Check sheet for the modelled part. Datum: model origin and axes. Units: mm. Coordinates: 2 decimals unless noted, no trailing zeros. Order: outer loops, then holes, each group sorted by start corner. A loop starts at its lowest first (then second) coordinate and runs counter-clockwise, first axis right, second up.
1. Gauge pin test, flat ends, axial feed: pin 1 Ø2.5 at (x, z) = (-43.3, -38.4) entering from -Y; pin 2 Ø1 at (x, y) = (76, 1) entering from -Z; pin 3 Ø6.5 at (x, z) = (56.5, 35.5) entering from +Y; pin 4 Ø1 at (x, y) = (14.5, 2.5) entering from +Z. Record the tip position at first contact, or that the pin passes through.
2. Draft check along X on faces 1 (the cylindrical face through (60.84, 1.52, -81.95)), 2 (the flat face through (1, 3, -11)), 3 (the conical face through (-51.97, 2.3, 55.43)). Enter one of: released by +X, released by -X, zero draft, split by the parting line, or undercut.
3. Cross-section at B-B (x = -69.5). Enter the section's corners in (y, z), then the cut area to 3 significant figures.
4. Cross-section at A-A (z = -63.5). Enter the section's corners in (x, y), then the cut area to 3 significant figures.
5. Thickness scan on line 1 (X direction, y = 0.3, z = 3.9); line 2 (X direction, y = 0.3, z = -22); line 3 (X direction, y = 0.3, z = -35.5). Record the ranges inside material, lowest first.
```python
from build123d import *

# Parameters (mm, degrees)
SKETCH1_R                                      = 100
BOSS_EXTRUDE1_DEPTH                            = 3
CSK_FOR_M5_SFHCS1_AT_2_COUNT                   = 2
CSK_FOR_M5_SFHCS1_AT_2_PITCH                   = 23.5
CSK_FOR_M5_SFHCS1_AT_3_COUNT                   = 2
CSK_FOR_M5_SFHCS1_AT_3_PITCH                   = 40.703193978
CSK_FOR_M5_SFHCS1_AT_4_COUNT                   = 2
CSK_FOR_M5_SFHCS1_AT_4_PITCH                   = 47
CSK_FOR_M5_SFHCS1_AT_5_COUNT                   = 2
CSK_FOR_M5_SFHCS1_AT_5_PITCH                   = 40.703193978
CSK_FOR_M5_SFHCS1_AT_6_COUNT                   = 2
CSK_FOR_M5_SFHCS1_AT_6_PITCH                   = 23.5
BOSS_EXTRUDE2_DEPTH                            = 3
FILLET1_R                                      = 20
CSK_FOR_M5_SFHCS2_AT_2_COUNT                   = 2
CSK_FOR_M5_SFHCS2_AT_2_PITCH                   = 35
CSK_FOR_M5_SFHCS2_AT_3_COUNT                   = 2
CSK_FOR_M5_SFHCS2_AT_3_PITCH                   = 45
CSK_FOR_M5_SFHCS2_AT_4_COUNT                   = 2
CSK_FOR_M5_SFHCS2_AT_4_PITCH                   = 57.008771255
CSK_FOR_M5_FLAT_HEAD_MACHINE_SCREW2_AT_2_COUNT = 2
CSK_FOR_M5_FLAT_HEAD_MACHINE_SCREW2_AT_2_PITCH = 70
CSK_FOR_M5_FLAT_HEAD_MACHINE_SCREW2_AT_3_COUNT = 2
CSK_FOR_M5_FLAT_HEAD_MACHINE_SCREW2_AT_3_PITCH = 99.704563587
CSK_FOR_M5_FLAT_HEAD_MACHINE_SCREW2_AT_4_COUNT = 2
CSK_FOR_M5_FLAT_HEAD_MACHINE_SCREW2_AT_4_PITCH = 71
CSK_FOR_M4_FLAT_HEAD_MACHINE_SCREW1_AT_2_COUNT = 2
CSK_FOR_M4_FLAT_HEAD_MACHINE_SCREW1_AT_2_PITCH = 42.3
CSK_FOR_M4_FLAT_HEAD_MACHINE_SCREW1_AT_3_COUNT = 2
CSK_FOR_M4_FLAT_HEAD_MACHINE_SCREW1_AT_3_PITCH = 40.4
CSK_FOR_M4_FLAT_HEAD_MACHINE_SCREW1_AT_4_COUNT = 2
CSK_FOR_M4_FLAT_HEAD_MACHINE_SCREW1_AT_4_PITCH = 58.493161994
CSK_FOR_M5_FLAT_HEAD_MACHINE_SCREW3_AT_2_COUNT = 2
CSK_FOR_M5_FLAT_HEAD_MACHINE_SCREW3_AT_2_PITCH = 155
CSK_FOR_M5_FLAT_HEAD_MACHINE_SCREW3_AT_3_COUNT = 2
CSK_FOR_M5_FLAT_HEAD_MACHINE_SCREW3_AT_3_PITCH = 109.601551084
CSK_FOR_M5_FLAT_HEAD_MACHINE_SCREW3_AT_4_COUNT = 2
CSK_FOR_M5_FLAT_HEAD_MACHINE_SCREW3_AT_4_PITCH = 109.601551084


with BuildPart() as part:
    # Sketch1 → Boss-Extrude1 (new body)
    with BuildSketch(Plane(origin=(0, 0, 0), x_dir=(1, 0, 0), z_dir=(0, 1, 0))):
        with Locations(Location((0, 0, 0), (0, 0, 270))):
            Circle(SKETCH1_R)
    extrude(amount=BOSS_EXTRUDE1_DEPTH)

    # Sketch6 → CSK for M5 SFHCS1 (revolve, cut)
    with BuildSketch(Plane(origin=(-13.325081846, 0, -19.356967578), x_dir=(0, 0, -1), z_dir=(1, 0, 0))):
        Polygon((0, 0), (0, 3), (2.65, 3), (2.65, 2.95), (5.6, 0), align=None)
    csk_for_m5_sfhcs1 = revolve(axis=Axis((-13.325081846, -6.35, -19.356967578), (0, 1, 0)), mode=Mode.SUBTRACT)

    # CSK for M5 SFHCS1 at 2: CSK for M5 SFHCS1 ×2
    with Locations(*[Vector(0.9968581525690036, 0, -0.07920747222777241) * (i * CSK_FOR_M5_SFHCS1_AT_2_PITCH) for i in range(1, CSK_FOR_M5_SFHCS1_AT_2_COUNT)]):
        add(csk_for_m5_sfhcs1, mode=Mode.SUBTRACT)

    # CSK for M5 SFHCS1 at 3: CSK for M5 SFHCS1 ×2
    with Locations(*[Vector(0.902908220208267, 0, 0.4298333931657005) * (i * CSK_FOR_M5_SFHCS1_AT_3_PITCH) for i in range(1, CSK_FOR_M5_SFHCS1_AT_3_COUNT)]):
        add(csk_for_m5_sfhcs1, mode=Mode.SUBTRACT)

    # CSK for M5 SFHCS1 at 4: CSK for M5 SFHCS1 ×2
    with Locations(*[Vector(0.5670247594033001, 0, 0.8237007479804968) * (i * CSK_FOR_M5_SFHCS1_AT_4_PITCH) for i in range(1, CSK_FOR_M5_SFHCS1_AT_4_COUNT)]):
        add(csk_for_m5_sfhcs1, mode=Mode.SUBTRACT)

    # CSK for M5 SFHCS1 at 5: CSK for M5 SFHCS1 ×2
    with Locations(*[Vector(0.07920747222776865, 0, 0.9968581525690039) * (i * CSK_FOR_M5_SFHCS1_AT_5_PITCH) for i in range(1, CSK_FOR_M5_SFHCS1_AT_5_COUNT)]):
        add(csk_for_m5_sfhcs1, mode=Mode.SUBTRACT)

    # CSK for M5 SFHCS1 at 6: CSK for M5 SFHCS1 ×2
    with Locations(*[Vector(-0.4298333931657009, 0, 0.9029082202082669) * (i * CSK_FOR_M5_SFHCS1_AT_6_PITCH) for i in range(1, CSK_FOR_M5_SFHCS1_AT_6_COUNT)]):
        add(csk_for_m5_sfhcs1, mode=Mode.SUBTRACT)

    # Sketch7 → Boss-Extrude2 (add)
    with BuildSketch(Plane.XZ):
        with BuildLine():
            Line((-16, -98.711701434), (-16, -180.1))
            Line((-16, -180.1), (59, -180.1))
            Line((59, -180.1), (59, -80.740324498))
            ThreePointArc((59, -80.740324498), (23.302201554, -97.247145988), (-16, -98.711701434))
        make_face()
    extrude(amount=-BOSS_EXTRUDE2_DEPTH)

    # Fillet1
    fillet1_edges = [part.edges().sort_by_distance(p)[0] for p in [
        (-16, 1.5, -98.711701434),
        (59, 1.5, -80.740324498),
        (59, 1.5, -180.1),
        (-16, 1.5, -180.1),
    ]]
    fillet(fillet1_edges, radius=FILLET1_R)

    # Sketch14 → CSK for M5 SFHCS2 (revolve, cut)
    with BuildSketch(Plane(origin=(39, 3, -160.1), x_dir=(0, 0, 1), z_dir=(1, 0, 0))):
        Polygon((0, 0), (0, 3), (2.65, 3), (2.65, 2.95), (5.6, 0), align=None)
    csk_for_m5_sfhcs2 = revolve(axis=Axis((39, 9.35, -160.1), (0, -1, 0)), mode=Mode.SUBTRACT)

    # CSK for M5 SFHCS2 at 2: CSK for M5 SFHCS2 ×2
    with Locations(*[(-i * CSK_FOR_M5_SFHCS2_AT_2_PITCH, 0, 0) for i in range(1, CSK_FOR_M5_SFHCS2_AT_2_COUNT)]):
        add(csk_for_m5_sfhcs2, mode=Mode.SUBTRACT)

    # CSK for M5 SFHCS2 at 3: CSK for M5 SFHCS2 ×2
    with Locations(*[(0, 0, i * CSK_FOR_M5_SFHCS2_AT_3_PITCH) for i in range(1, CSK_FOR_M5_SFHCS2_AT_3_COUNT)]):
        add(csk_for_m5_sfhcs2, mode=Mode.SUBTRACT)

    # CSK for M5 SFHCS2 at 4: CSK for M5 SFHCS2 ×2
    with Locations(*[Vector(-0.6139406135149205, 0, 0.7893522173763264) * (i * CSK_FOR_M5_SFHCS2_AT_4_PITCH) for i in range(1, CSK_FOR_M5_SFHCS2_AT_4_COUNT)]):
        add(csk_for_m5_sfhcs2, mode=Mode.SUBTRACT)

    # Sketch17 → CSK for M5 Flat Head Machine Screw2 (revolve, cut)
    with BuildSketch(Plane(origin=(56.5, 3, -35.5), x_dir=(0, 0, 1), z_dir=(1, 0, 0))):
        Polygon((0, 0), (0, 3), (2.75, 3), (2.75, 2.45), (5.2, 0), align=None)
    csk_for_m5_flat_head_machine_screw2 = revolve(axis=Axis((56.5, 9.35, -35.5), (0, -1, 0)), mode=Mode.SUBTRACT)

    # CSK for M5 Flat Head Machine Screw2 at 2: CSK for M5 Flat Head Machine Screw2 ×2
    with Locations(*[(-i * CSK_FOR_M5_FLAT_HEAD_MACHINE_SCREW2_AT_2_PITCH, 0, 0) for i in range(1, CSK_FOR_M5_FLAT_HEAD_MACHINE_SCREW2_AT_2_COUNT)]):
        add(csk_for_m5_flat_head_machine_screw2, mode=Mode.SUBTRACT)

    # CSK for M5 Flat Head Machine Screw2 at 3: CSK for M5 Flat Head Machine Screw2 ×2
    with Locations(*[Vector(-0.7020741827848285, 0, 0.7121038139674688) * (i * CSK_FOR_M5_FLAT_HEAD_MACHINE_SCREW2_AT_3_PITCH) for i in range(1, CSK_FOR_M5_FLAT_HEAD_MACHINE_SCREW2_AT_3_COUNT)]):
        add(csk_for_m5_flat_head_machine_screw2, mode=Mode.SUBTRACT)

    # CSK for M5 Flat Head Machine Screw2 at 4: CSK for M5 Flat Head Machine Screw2 ×2
    with Locations(*[(0, 0, i * CSK_FOR_M5_FLAT_HEAD_MACHINE_SCREW2_AT_4_PITCH) for i in range(1, CSK_FOR_M5_FLAT_HEAD_MACHINE_SCREW2_AT_4_COUNT)]):
        add(csk_for_m5_flat_head_machine_screw2, mode=Mode.SUBTRACT)

    # Sketch19 → CSK for M4 Flat Head Machine Screw1 (revolve, cut)
    with BuildSketch(Plane(origin=(-43.3, 3, -38.4), x_dir=(0, 0, 1), z_dir=(1, 0, 0))):
        Polygon((0, 0), (0, 3), (2.25, 3), (2.25, 2.45), (4.7, 0), align=None)
    csk_for_m4_flat_head_machine_screw1 = revolve(axis=Axis((-43.3, 9.35, -38.4), (0, -1, 0)), mode=Mode.SUBTRACT)

    # CSK for M4 Flat Head Machine Screw1 at 2: CSK for M4 Flat Head Machine Screw1 ×2
    with Locations(*[(0, 0, i * CSK_FOR_M4_FLAT_HEAD_MACHINE_SCREW1_AT_2_PITCH) for i in range(1, CSK_FOR_M4_FLAT_HEAD_MACHINE_SCREW1_AT_2_COUNT)]):
        add(csk_for_m4_flat_head_machine_screw1, mode=Mode.SUBTRACT)

    # CSK for M4 Flat Head Machine Screw1 at 3: CSK for M4 Flat Head Machine Screw1 ×2
    with Locations(*[(-i * CSK_FOR_M4_FLAT_HEAD_MACHINE_SCREW1_AT_3_PITCH, 0, 0) for i in range(1, CSK_FOR_M4_FLAT_HEAD_MACHINE_SCREW1_AT_3_COUNT)]):
        add(csk_for_m4_flat_head_machine_screw1, mode=Mode.SUBTRACT)

    # CSK for M4 Flat Head Machine Screw1 at 4: CSK for M4 Flat Head Machine Screw1 ×2
    with Locations(*[Vector(-0.6906790233784355, 0, 0.7231614526957384) * (i * CSK_FOR_M4_FLAT_HEAD_MACHINE_SCREW1_AT_4_PITCH) for i in range(1, CSK_FOR_M4_FLAT_HEAD_MACHINE_SCREW1_AT_4_COUNT)]):
        add(csk_for_m4_flat_head_machine_screw1, mode=Mode.SUBTRACT)

    # Sketch21 → CSK for M5 Flat Head Machine Screw3 (revolve, cut)
    with BuildSketch(Plane(origin=(-54.800775542, 0, 54.800775542), x_dir=(0, 0, -1), z_dir=(1, 0, 0))):
        Polygon((0, 0), (0, 3), (2.75, 3), (2.75, 2.45), (5.2, 0), align=None)
    csk_for_m5_flat_head_machine_screw3 = revolve(axis=Axis((-54.800775542, -6.35, 54.800775542), (0, 1, 0)), mode=Mode.SUBTRACT)

    # CSK for M5 Flat Head Machine Screw3 at 2: CSK for M5 Flat Head Machine Screw3 ×2
    with Locations(*[Vector(0.7071067811865415, 0, -0.7071067811865537) * (i * CSK_FOR_M5_FLAT_HEAD_MACHINE_SCREW3_AT_2_PITCH) for i in range(1, CSK_FOR_M5_FLAT_HEAD_MACHINE_SCREW3_AT_2_COUNT)]):
        add(csk_for_m5_flat_head_machine_screw3, mode=Mode.SUBTRACT)

    # CSK for M5 Flat Head Machine Screw3 at 3: CSK for M5 Flat Head Machine Screw3 ×2
    with Locations(*[(0, 0, -i * CSK_FOR_M5_FLAT_HEAD_MACHINE_SCREW3_AT_3_PITCH) for i in range(1, CSK_FOR_M5_FLAT_HEAD_MACHINE_SCREW3_AT_3_COUNT)]):
        add(csk_for_m5_flat_head_machine_screw3, mode=Mode.SUBTRACT)

    # CSK for M5 Flat Head Machine Screw3 at 4: CSK for M5 Flat Head Machine Screw3 ×2
    with Locations(*[(i * CSK_FOR_M5_FLAT_HEAD_MACHINE_SCREW3_AT_4_PITCH, 0, 0) for i in range(1, CSK_FOR_M5_FLAT_HEAD_MACHINE_SCREW3_AT_4_COUNT)]):
        add(csk_for_m5_flat_head_machine_screw3, mode=Mode.SUBTRACT)


solid = part.part
```
Data:
1. pin 1: passes through
1. pin 2: stops at z = -65.57
1. pin 3: stops at y = 1.05
1. pin 4: stops at z = 99.02
2. face 1: released by +X
2. face 2: zero draft
2. face 3: undercut
3. outline: (0, -71.9) - (3, -71.9) - (3, 71.9) - (0, 71.9) - close
3. area: 431 mm2
4. outline: (-77.25, 0) - (77.25, 0) - (77.25, 3) - (-77.25, 3) - close
4. area: 464 mm2
5. line 1: x = -99.92 to -85.95, -81.45 to -45.55, -41.05 to -28.32, -18.53 to 99.92
5. line 2: x = -97.55 to -17.92, -8.73 to 4.86, 15.34 to 97.55
5. line 3: x = -93.49 to -16.25, -10.75 to 53.75, 59.25 to 93.49
